Check sheet for the modelled part. Datum: model origin and axes. Units: mm. Face numbers are marked on the shaded views. A direction names the side the tool comes from. Give positions to 0.01 mm unless a question says otherwise; leave off trailing zeros. Loops run counter-clockwise (first coordinate to the right, second up) from the corner with the lowest first, then second, coordinate; pieces in that order, holes last.
```python
from build123d import *

# Parameters (mm, degrees)
EXTRUDE_1_DEPTH     = 1.6
EXTRUDE_2_DEPTH     = 2
CUT_EXTRUDE_1_DEPTH = 3.1
CUT_EXTRUDE_2_DEPTH = 1


with BuildPart() as part:
    # 草图1 → 凸台-拉伸1 (new body)
    with BuildSketch(Plane(origin=(0, 0, 0), x_dir=(1, 0, 0), z_dir=(0, 1, 0))):
        with BuildLine():
            Line((-3.8, 4.8), (3.8, 4.8))
            ThreePointArc((3.8, 4.8), (4.507106781, 4.507106781), (4.8, 3.8))
            Line((4.8, 3.8), (4.8, -3.8))
            ThreePointArc((4.8, -3.8), (4.507106781, -4.507106781), (3.8, -4.8))
            Line((3.8, -4.8), (-3.8, -4.8))
            ThreePointArc((-3.8, -4.8), (-4.507106781, -4.507106781), (-4.8, -3.8))
            Line((-4.8, -3.8), (-4.8, 3.8))
            ThreePointArc((-4.8, 3.8), (-4.507106781, 4.507106781), (-3.8, 4.8))
        make_face()
    extrude(amount=EXTRUDE_1_DEPTH)

    # 草图2 → 凸台-拉伸2 (add)
    with BuildSketch(Plane.XZ):
        with BuildLine():
            Line((-5.6, 6.6), (5.6, 6.6))
            ThreePointArc((5.6, 6.6), (6.307106781, 6.307106781), (6.6, 5.6))
            Line((6.6, 5.6), (6.6, -5.6))
            ThreePointArc((6.6, -5.6), (6.307106781, -6.307106781), (5.6, -6.6))
            Line((5.6, -6.6), (-5.6, -6.6))
            ThreePointArc((-5.6, -6.6), (-6.307106781, -6.307106781), (-6.6, -5.6))
            Line((-6.6, -5.6), (-6.6, 5.6))
            ThreePointArc((-6.6, 5.6), (-6.307106781, 6.307106781), (-5.6, 6.6))
        make_face()
    extrude(amount=EXTRUDE_2_DEPTH)

    # 草图3 → 切除-拉伸1 (cut)
    with BuildSketch(Plane.XZ.offset(2)):
        with BuildLine():
            Line((-3.3, -4.3), (3.3, -4.3))
            ThreePointArc((3.3, -4.3), (4.007106781, -4.007106781), (4.3, -3.3))
            Line((4.3, -3.3), (4.3, 3.3))
            ThreePointArc((4.3, 3.3), (4.007106781, 4.007106781), (3.3, 4.3))
            Line((3.3, 4.3), (-3.3, 4.3))
            ThreePointArc((-3.3, 4.3), (-4.007106781, 4.007106781), (-4.3, 3.3))
            Line((-4.3, 3.3), (-4.3, -3.3))
            ThreePointArc((-4.3, -3.3), (-4.007106781, -4.007106781), (-3.3, -4.3))
        make_face()
    extrude(amount=-CUT_EXTRUDE_1_DEPTH, mode=Mode.SUBTRACT)

    # 草图4 → 切除-拉伸2 (cut)
    with BuildSketch(Plane.XZ.offset(2)):
        with BuildLine():
            Line((-4.6, 5.6), (4.6, 5.6))
            ThreePointArc((4.6, 5.6), (5.307106781, 5.307106781), (5.6, 4.6))
            Line((5.6, 4.6), (5.6, -4.6))
            ThreePointArc((5.6, -4.6), (5.307106781, -5.307106781), (4.6, -5.6))
            Line((4.6, -5.6), (-4.6, -5.6))
            ThreePointArc((-4.6, -5.6), (-5.307106781, -5.307106781), (-5.6, -4.6))
            Line((-5.6, -4.6), (-5.6, 4.6))
            ThreePointArc((-5.6, 4.6), (-5.307106781, 5.307106781), (-4.6, 5.6))
        make_face()
    extrude(amount=-CUT_EXTRUDE_2_DEPTH, mode=Mode.SUBTRACT)


solid = part.part
```
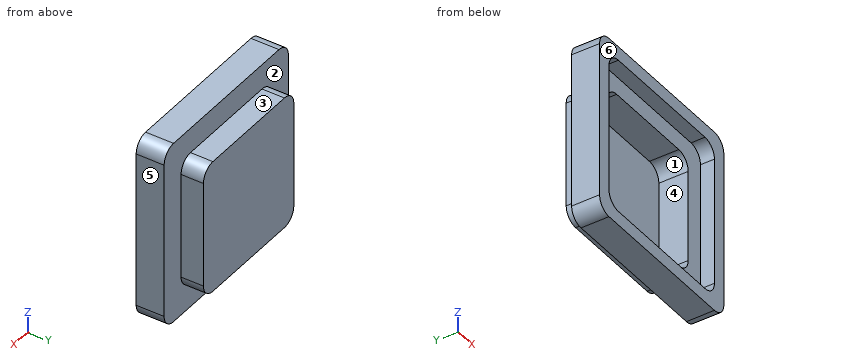
(1) Release check for a two-part mould opening along X. For the marked faces 4, 5 and 6 record: pulls with the +X half, pulls with the -X half, needs draft (parallel to the pull), parting line crosses it, or undercut.
(2) Access from +Z, -Z, +X, -X, +Y, -Y to the whole of each face (thin tool, end or side, straight path). Record for the marked faces 1, 2 and 3.
(3) Section check D-D on y = -0.2. Record the boundary of the cut face in (x, z), plus the area to 3 significant figures.
(4) Material ranges on line 1 (Z direction, x = -0.5, y = -0.6); line 2 (Z direction, x = -2.5, y = 0.1); line 3 (X direction, y = -1.6, z = -4.25), recorded low to high.
(5) Section check C-C on z = 1.5. Record the boundary of the cut face in (x, y).
(6) Gauge pin test, flat ends, axial feed: pin 1 Ø4 at (x, z) = (-3.5, -2) entering from -Y; pin 2 Ø0.8 at (x, y) = (-1.5, 0.5) entering from -Z; pin 3 Ø1.8 at (y, z) = (1, -1) entering from -X. Record the tip position at first contact, or that the pin passes through.
(7) Section check B-B on x = 0. Record the boundary of the cut face in (y, z).
(8) Section check A-A on y = -1.55. Record the boundary of the cut face in (x, z).
Computed values:
1. face 4: undercut
1. face 5: pulls with the +X half
1. face 6: needs draft
2. face 1: -Y
2. face 2: +Y
2. face 3: +Z, +X, -X, +Y
3. outline: (-6.6, -5.6) arc R1 ccw to (-5.6, -6.6) - (5.6, -6.6) arc R1 ccw to (6.6, -5.6) - (6.6, 5.6) arc R1 ccw to (5.6, 6.6) - (-5.6, 6.6) arc R1 ccw to (-6.6, 5.6) - close; hole (-4.3, -3.3) arc R1 ccw to (-3.3, -4.3) - (3.3, -4.3) arc R1 ccw to (4.3, -3.3) - (4.3, 3.3) arc R1 ccw to (3.3, 4.3) - (-3.3, 4.3) arc R1 ccw to (-4.3, 3.3) - close
3. area: 100 mm2
4. line 1: z = -6.6 to -4.3, 4.3 to 6.6
4. line 2: z = -4.8 to -4.3, 4.3 to 4.8
4. line 3: x = -6.6 to -5.6, 5.6 to 6.6
5. outline: (-6.6, -2) - (-5.6, -2) - (-5.6, -1) - (-4.3, -1) - (-4.3, 1.1) - (4.3, 1.1) - (4.3, -1) - (5.6, -1) - (5.6, -2) - (6.6, -2) - (6.6, 0) - (4.8, 0) - (4.8, 1.6) - (-4.8, 1.6) - (-4.8, 0) - (-6.6, 0) - close
6. pin 1: stops at y = -1
6. pin 2: stops at z = -4.8
6. pin 3: stops at x = -4.8
7. outline: (-2, -6.6) - (0, -6.6) - (0, -4.8) - (1.6, -4.8) - (1.6, 4.8) - (0, 4.8) - (0, 6.6) - (-2, 6.6) - (-2, 5.6) - (-1, 5.6) - (-1, 4.3) - (1.1, 4.3) - (1.1, -4.3) - (-1, -4.3) - (-1, -5.6) - (-2, -5.6) - close
8. outline: (-6.6, -5.6) arc R1 ccw to (-5.6, -6.6) - (5.6, -6.6) arc R1 ccw to (6.6, -5.6) - (6.6, 5.6) arc R1 ccw to (5.6, 6.6) - (-5.6, 6.6) arc R1 ccw to (-6.6, 5.6) - close; hole (-5.6, -4.6) arc R1 ccw to (-4.6, -5.6) - (4.6, -5.6) arc R1 ccw to (5.6, -4.6) - (5.6, 4.6) arc R1 ccw to (4.6, 5.6) - (-4.6, 5.6) arc R1 ccw to (-5.6, 4.6) - close
